Design review of the part built by this model. Coordinates are the model's own, in mm. Face numbers are marked on the shaded views. A direction names the side the tool comes from. Round coordinates to 2 decimals unless told otherwise and drop trailing zeros. Write each loop counter-clockwise with the first axis right and the second up, starting at its lowest first coordinate (ties: lowest second). Pieces come first, ordered by that corner, then holes.
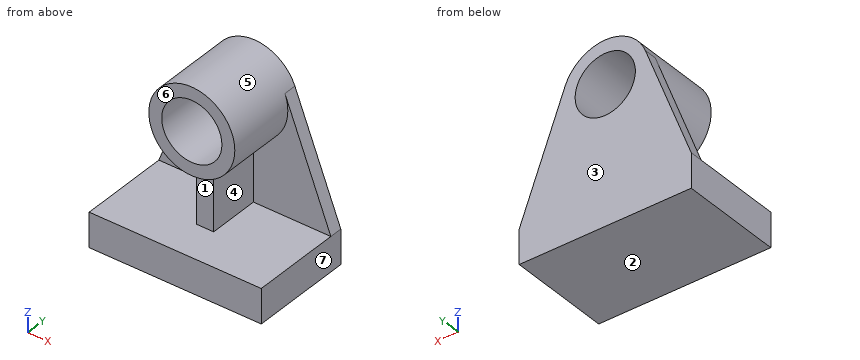
from build123d import *

# Parameters (mm, degrees)
F0_R     = 44.45
F1_DEPTH = 19.05
F2_W     = 254
F2_H     = 50.8
F3_DEPTH = 133.35
F4_R     = 63.5
F4_R_2   = 44.45
F5_DEPTH = 101.6
F7_DEPTH = 76.2


with BuildPart() as f1:
    # F0 (on Front) → F1 (new body)
    with BuildSketch(Plane.XZ):
        with BuildLine():
            Line((-137.7003500163, 50.8), (-137.7003500163, 0))
            Line((-137.7003500163, 0), (116.2996499837, 0))
            Line((116.2996499837, 0), (116.2996499837, 50.8))
            Line((116.2996499837, 50.8), (48.5273968003, 226.0981223472))
            ThreePointArc((48.5273968003, 226.0981223472), (-10.7003500163, 266.7), (-69.9280968329, 226.0981223472))
            Line((-69.9280968329, 226.0981223472), (-137.7003500163, 50.8))
        make_face()
        with Locations((-10.7003500163, 203.2)):
            Circle(F0_R, mode=Mode.SUBTRACT)
    extrude(amount=F1_DEPTH)

    # F2 (on face) → F3 (join)
    with BuildSketch(Plane.XZ.offset(19.05)):
        with Locations((-10.7003500163, 25.4)):
            Rectangle(F2_W, F2_H)
    extrude(amount=F3_DEPTH)

    # F4 (on face) → F5 (join)
    with BuildSketch(Plane.XZ.offset(19.05)):
        with Locations((-10.7003500163, 203.2)):
            Circle(F4_R)
        with Locations((-10.7003500163, 203.2)):
            Circle(F4_R_2, mode=Mode.SUBTRACT)
    extrude(amount=F5_DEPTH)

    # F6 (on face) → F7 (join)
    with BuildSketch(Plane.XZ.offset(19.05)):
        with BuildLine():
            Line((1.9996499837, 50.8), (1.9996499837, 140.9829605333))
            ThreePointArc((1.9996499837, 140.9829605333), (-10.7003500163, 139.7), (-23.4003500163, 140.9829605333))
            Line((-23.4003500163, 140.9829605333), (-23.4003500163, 50.8))
            Line((-23.4003500163, 50.8), (1.9996499837, 50.8))
        make_face()
    extrude(amount=F7_DEPTH)


solid = f1.part
1) For P1, Ø7.5, axis at x = -9.5, z = 82, coming from the -Y side; P2, Ø4, axis at x = 56, z = 216, coming from the -Y side, all flat-tipped, find the tip position at first contact; note any pin that passes through.
2) For line 1 along Z through (x, y) = (-13.5, -143.5); line 2 along Y through (x, z) = (17.5, 122); line 3 along X through (y, z) = (-25.5, 193.5), list the stretches that pass through material, from the lowest coordinate up.
3) Add section C-C on z = 196.5. State the section outline as (x, y) points, and give its area (3 significant figures).
4) Add section B-B on x = -15.5. State the section outline as (y, z) points.
5) The part is to be moulded in two halves that separate along Z. For the marked faces 1, 2 and 3, say which applies: pulls with the +Z half, pulls with the -Z half, needs draft (parallel to the pull), parting line crosses it, or undercut.
6) Add section A-A on y = -15. State the section outline as (x, z) points.
7) Add section D-D on y = -38.5. State the section outline as (x, z) points, and give its area (3 significant figures).
8) For the marked faces 4, 5, 6 and 7, list the 3-axis set-ups (+Z, -Z, +X, -X, +Y, -Y) from which the entire face can be reached by the end or side of a thin tool; tool diameter is ignored.
Computed:
1. P1: stops at y = -95.25
1. P2: passes through
2. line 1: z = 0 to 50.8
2. line 2: y = -19.05 to 0
2. line 3: x = -73.46 to -54.08, 32.68 to 52.05
3. outline: (-81.37, -19.05) - (-73.85, -19.05) - (-73.85, -120.65) - (-54.64, -120.65) - (-54.64, 0) - (-81.37, 0) - close; (33.24, -120.65) - (52.45, -120.65) - (52.45, -19.05) - (59.97, -19.05) - (59.97, 0) - (33.24, 0) - close
3. area: 4,920 mm2
4. outline: (-152.4, 0) - (0, 0) - (0, 159.01) - (-120.65, 159.01) - (-120.65, 139.88) - (-95.25, 139.88) - (-95.25, 50.8) - (-152.4, 50.8) - close; (-120.65, 247.39) - (0, 247.39) - (0, 266.52) - (-120.65, 266.52) - close
5. face 1: undercut
5. face 2: pulls with the -Z half
5. face 3: needs draft
6. outline: (-137.7, 0) - (116.3, 0) - (116.3, 50.8) - (48.53, 226.1) arc R63.5 ccw to (-69.93, 226.1) - (-137.7, 50.8) - close; hole circle Ø88.9 at (-10.7, 203.2)
7. outline: (-137.7, 0) - (116.3, 0) - (116.3, 50.8) - (2, 50.8) - (2, 140.98) arc R63.5 ccw (long way) to (-23.4, 140.98) - (-23.4, 50.8) - (-137.7, 50.8) - close; hole circle Ø88.9 at (-10.7, 203.2)
7. area: 21,600 mm2
8. face 4: +X, -Y
8. face 5: -Y
8. face 6: +Z, +X, -X, -Y
8. face 7: +Z, -Z, +X, +Y, -Y
